Design review of the part built by this model. Coordinates are the model's own, in mm. Face numbers are marked on the shaded views. A direction names the side the tool comes from. Coordinates: 2 decimals unless noted, no trailing zeros. Order: outer loops, then holes, each group sorted by start corner. A loop starts at its lowest first (then second) coordinate and runs counter-clockwise, first axis right, second up. Notation, with made-up numbers: M -17,-23.75 L 18,-23.75 A11 cw 18,-16.75 Z; hole C 20.25,-35.75 d4. An arc over 180 degrees is marked long. Answer in a Markdown table with one row per item.
from build123d import *

# Parameters (mm, degrees)
F0_W     = 15
F0_H     = 25
F1_DEPTH = 4
F3_DEPTH = 8
F5_DEPTH = 4
F6_R     = 5


# Not quite as in the source:
# - a feature names something its author has since deleted; it is built from what else it names


with BuildPart() as f1:
    # F0 (on Top) → F1 (new body)
    with BuildSketch(Plane.XY):
        with Locations((38.2812308715, -12.5)):
            Rectangle(F0_W, F0_H)
    extrude(amount=F1_DEPTH)

    # F2 (on face) → F3 (join)
    with BuildSketch(Plane(origin=(30.7812308715, 0, 0), x_dir=(0, -1, 0), z_dir=(-1, 0, 0))):
        Polygon((13.6547005384, 0), (14.8094010768, 2), (13.6547005384, 4), (11.3452994616, 4), (10.1905989232, 2), (11.3452994616, 0), align=None)
    extrude(amount=F3_DEPTH)

    # F4 (on face) → F5 (cut, through all)
    with BuildSketch(Plane.XY.offset(4)):
        with BuildLine():
            Line((34.7812308715, -16.5), (41.7812308715, -16.5))
            ThreePointArc((41.7812308715, -16.5), (38.2812308715, -13), (34.7812308715, -16.5))
        make_face()
        with BuildLine():
            ThreePointArc((34.7812308715, -16.5), (38.2812308715, -20), (41.7812308715, -16.5))
            Line((41.7812308715, -16.5), (34.7812308715, -16.5))
        make_face()
        with BuildLine():
            ThreePointArc((34.7812308715, -16.5), (38.2812308715, -13), (41.7812308715, -16.5))
            Line((41.7812308715, -16.5), (41.7812308715, -8.5))
            ThreePointArc((41.7812308715, -8.5), (38.2812308715, -12), (34.7812308715, -8.5))
            Line((34.7812308715, -8.5), (34.7812308715, -16.5))
        make_face()
        with BuildLine():
            Line((34.7812308715, -8.5), (41.7812308715, -8.5))
            ThreePointArc((41.7812308715, -8.5), (38.2812308715, -5), (34.7812308715, -8.5))
        make_face()
        with BuildLine():
            ThreePointArc((34.7812308715, -8.5), (38.2812308715, -12), (41.7812308715, -8.5))
            Line((41.7812308715, -8.5), (34.7812308715, -8.5))
        make_face()
    extrude(amount=-F5_DEPTH, mode=Mode.SUBTRACT)

    # F6
    f6_edges = [f1.edges().sort_by_distance(p)[0] for p in [
        (45.781231, 0, 2),
        (30.781231, 0, 2),
        (45.781231, -25, 2),
        (30.781231, -25, 2),
    ]]
    fillet(f6_edges, radius=F6_R)


solid = f1.part
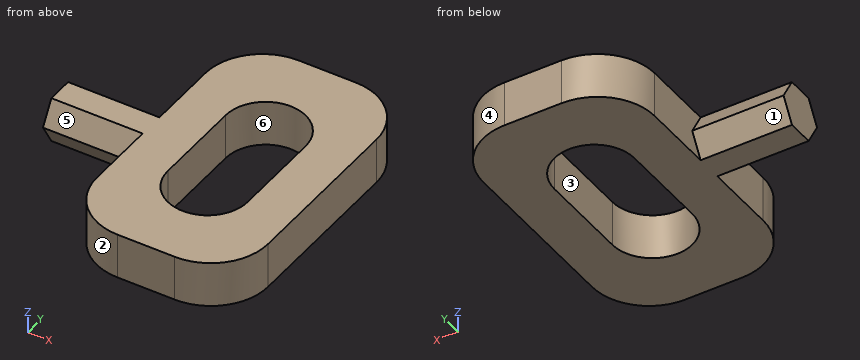
(1) Draft analysis for pull direction Y (two halves, no side actions). For the marked faces 1, 2 and 3, state which applies: pulls with the +Y half, pulls with the -Y half, needs draft (parallel to the pull), parting line crosses it, or undercut.
Return value:
| item | result |
|---|---|
| face 1 | pulls with the +Y half |
| face 2 | pulls with the -Y half |
| face 3 | undercut |
(2) For the marked faces 4, 5 and 6, list the 3-axis set-ups (+Z, -Z, +X, -X, +Y, -Y) from which the entire face can be reached by the end or side of a thin tool; tool diameter is ignored.
Return value:
| item | result |
|---|---|
| face 4 | +Z, -Z, +X, +Y |
| face 5 | +Z, -X, -Y |
| face 6 | +Z, -Z |
(3) Insertion check: pin 1 Ø2 at (y, z) = (-6.5, 3) entering from -X; pin 2 Ø1.5 at (x, z) = (42, 1) entering from +Y. Each pin has a flat end and moves straight along its axis. Give the tip position at first contact, or say it passes through.
Return value:
| item | result |
|---|---|
| pin 1 | stops at x = 30.78 |
| pin 2 | stops at y = -0.02 |
(4) Add section B-B, the plane y = -19. Give the boundary of the cut face in (x, z), and give its area (3 significant figures).
Return value:
| item | result |
|---|---|
| outline | M 30.78,0 L 35.83,0 L 35.83,4 L 30.78,4 Z; M 40.73,0 L 45.78,0 L 45.78,4 L 40.73,4 Z |
| area | 40.4 mm2 |
(5) Add section A-A, the plane z = 1. Give the boundary of the cut face in (x, y).
Return value:
| item | result |
|---|---|
| outline | M 22.78,-14.23 L 30.78,-14.23 L 30.78,-20 A5 ccw 35.78,-25 L 40.78,-25 A5 ccw 45.78,-20 L 45.78,-5 A5 ccw 40.78,0 L 35.78,0 A5 ccw 30.78,-5 L 30.78,-10.77 L 22.78,-10.77 Z; hole M 34.78,-16.5 A3.5 ccw 41.78,-16.5 L 41.78,-8.5 A3.5 ccw 34.78,-8.5 Z |
(6) Add section D-D, the plane x = 36.25. Give the boundary of the cut face in (y, z).
Return value:
| item | result |
|---|---|
| outline | M -25,0 L -19.35,0 L -19.35,4 L -25,4 Z; M -5.65,0 L 0,0 L 0,4 L -5.65,4 Z |
(7) Add section C-C, the plane x = 28.5. Give the boundary of the cut face in (y, z).
Return value:
| item | result |
|---|---|
| outline | M -14.81,2 L -13.65,0 L -11.35,0 L -10.19,2 L -11.35,4 L -13.65,4 Z |
(8) For line 1 along X through (y, z) = (-9, 1.15); line 2 along X through (y, z) = (-13.25, 3.6); line 3 along Y through (x, z) = (37.75, 3.4), list the stretches that pass through material, from the lowest coordinate up. Write a range as from..to.
Return value:
| item | result |
|---|---|
| line 1 | x = 30.78..34.78, 41.78..45.78 |
| line 2 | x = 22.78..34.78, 41.78..45.78 |
| line 3 | y = -25..-19.96, -5.04..0 |
